from build123d import *

# Parameters (mm, degrees)
F0_R           = 3.75
F1_DEPTH       = 1
F2_R           = 5
F3_R           = 1
F5_DEPTH       = 25
F7_DEPTH       = 25
F8_T1_DEPTH    = 10.2705098312
F10_DEPTH      = 30
F10_DEPTH_BACK = 25


# Not quite as in the source:
# - a fillet or chamfer that OpenCascade refuses, or shapes differently, is made with other operations: its cross-section is extruded or revolved along the edge and cut away or added


with BuildPart() as f1:
    # F0 (on Front) → F1 (new body)
    with BuildSketch(Plane.XZ):
        with BuildLine():
            Line((-27.5, -10), (7.9370479853, -10))
            Line((7.9370479853, -10), (20.3712052174, -7.3570382915))
            ThreePointArc((20.3712052174, -7.3570382915), (25.1669262461, -4.5995427), (27.4438066413, 0.4421373561))
            ThreePointArc((27.4438066413, 0.4421373561), (27.487512587, 1.2231450576), (27.4438066413, 2.004152759))
            ThreePointArc((27.4438066413, 2.004152759), (24.4984425132, 7.7095966656), (18.5, 10))
            Line((18.5, 10), (-12.5, 10))
            Line((-12.5, 10), (-27.5, -10))
        make_face()
        with Locations((18.5, 1.2231450576)):
            Circle(F0_R, mode=Mode.SUBTRACT)
    extrude(amount=F1_DEPTH)

    # F2
    f2_edges = [f1.edges().sort_by_distance(p)[0] for p in [
        (-12.5, -0.5, 10),
    ]]
    fillet(f2_edges, radius=F2_R)

    # F3
    f3_edges = [f1.edges().sort_by_distance(p)[0] for p in [
        (-27.5, -0.5, -10),
    ]]
    fillet(f3_edges, radius=F3_R)

    # F4 (on face) → F5 (cut)
    with BuildSketch(Plane.XZ.offset(1)):
        Polygon((-24.7211863589, -8.9615818119), (-25.5, -10), (-25.5, -14.0343736857), (7.9370479853, -14.0343736857), (8.0576272821, -10), (7.2788136411, -8.9615818119), (6.5, -10), (6.4576272821, -10), (5.6788136411, -8.9615818119), (4.9, -10), (4.8576272821, -10), (4.0788136411, -8.9615818119), (3.3, -10), (3.2576272821, -10), (2.4788136411, -8.9615818119), (1.7, -10), (1.6576272821, -10), (0.8788136411, -8.9615818119), (0.1, -10), (0.0576272821, -10), (-0.7211863589, -8.9615818119), (-1.5, -10), (-1.5423727179, -10), (-2.3211863589, -8.9615818119), (-3.1, -10), (-3.1423727179, -10), (-3.9211863589, -8.9615818119), (-4.7, -10), (-4.7423727179, -10), (-5.5211863589, -8.9615818119), (-6.3, -10), (-6.3423727179, -10), (-7.1211863589, -8.9615818119), (-7.9, -10), (-7.9423727179, -10), (-8.7211863589, -8.9615818119), (-9.5, -10), (-9.5423727179, -10), (-10.3211863589, -8.9615818119), (-11.1, -10), (-11.1423727179, -10), (-11.9211863589, -8.9615818119), (-12.7, -10), (-12.7423727179, -10), (-13.5211863589, -8.9615818119), (-14.3, -10), (-14.3423727179, -10), (-15.1211863589, -8.9615818119), (-15.9, -10), (-15.9423727179, -10), (-16.7211863589, -8.9615818119), (-17.5, -10), (-17.5423727179, -10), (-18.3211863589, -8.9615818119), (-19.1, -10), (-19.1423727179, -10), (-19.9211863589, -8.9615818119), (-20.7, -10), (-20.7423727179, -10), (-21.5211863589, -8.9615818119), (-22.3, -10), (-22.3423727179, -10), (-23.1211863589, -8.9615818119), (-23.9, -10), (-23.9423727179, -10), align=None)
    extrude(amount=-F5_DEPTH, mode=Mode.SUBTRACT)

    # F6 (on face) → F7 (cut)
    with BuildSketch(Plane.XZ.offset(1)):
        Polygon((-26.6561899334, -14.2840119079), (-25.5, -10), (-26.3, -8.4), (-30.4410159588, -7.8742252663), align=None)
    extrude(amount=-F7_DEPTH, mode=Mode.SUBTRACT)

    # F8: fillet of radius 3 on 1 edges, made by hand

    # F8_s2 → F8_t1 (cut)
    with BuildSketch(Plane.XZ.offset(-4.6352549156)):
        with BuildLine():
            ThreePointArc((-25.1875388203, -6.916718427), (-25.7754167621, -8.4473016411), (-25.4708203932, -10.0583592135))
            Line((-25.4708203932, -10.0583592135), (-26.3, -8.4))
            Line((-26.3, -8.4), (-25.1875388203, -6.916718427))
        make_face()
    extrude(amount=F8_T1_DEPTH, mode=Mode.SUBTRACT)

    # F9 (on Right) → F10 (cut, two sides)
    with BuildSketch(Plane.YZ) as f10_sk:
        Polygon((-2.5567745324, -10.8186043799), (-0.4, -10), (-1, -6.9173601342), (-2.5567745324, -6.9173601342), align=None)
    extrude(amount=-F10_DEPTH, mode=Mode.SUBTRACT)
    extrude(f10_sk.sketch, amount=F10_DEPTH_BACK, mode=Mode.SUBTRACT)


solid = f1.part
For this review, take the finished solid that the model builds, in its own axes (mm). Round coordinates to 2 decimals unless told otherwise and drop trailing zeros. Write each loop counter-clockwise with the first axis right and the second up, starting at its lowest first coordinate (ties: lowest second). Pieces come first, ordered by that corner, then holes. Notation, with made-up numbers: (86, 89) - (101, 89) arc R33 cw to (101, 126) - close; hole circle Ø5 at (-34.75, 87). An arc over 180 degrees is marked (long way). Use a Markdown table: item, result.
Q1. We need section B-B (x = 17). Give the boundary of the cut face in (y, z).
Derived:
| item | result |
|---|---|
| outline | (-1, -6.92) - (-0.77, -8.07) - (0, -8.07) - (0, -2.21) - (-1, -2.21) - close; (-1, 4.66) - (0, 4.66) - (0, 10) - (-1, 10) - close |
Q2. We need section A-A (z = 3.5). Give the boundary of the cut face in (x, y) (3 decimals), plus the area to 3 significant figures.
Derived:
| item | result |
|---|---|
| outline | (-17.375, -1) - (15.52, -1) - (15.52, 0) - (-17.375, 0) - close; (21.48, -1) - (27.146, -1) - (27.146, 0) - (21.48, 0) - close |
| area | 38.6 mm2 |
Q3. The part is to be moulded in two halves that separate along X. For faces 1 (the cylindrical face through (14.754, -0.493, 1.388)), 2 (the flat face through (0, 0, 0)), 3 (the cylindrical face through (25.11, -0.49, -4.66)), say which applies: pulls with the +X half, pulls with the -X half, needs draft (parallel to the pull), parting line crosses it, or undercut.
Derived:
| item | result |
|---|---|
| face 1 | undercut |
| face 2 | needs draft |
| face 3 | pulls with the +X half |
Q4. Wall thickness on line 1 along X through (y, z) = (-0.35, 4.25); line 2 along Z through (x, y) = (18.5, -0.55); line 3 along X through (y, z) = (-0.65, 0): over which ranges is each line inside the solid? List them lowest first.
Derived:
| item | result |
|---|---|
| line 1 | x = -16.81 to 16.29, 20.71 to 26.89 |
| line 2 | z = -7.75 to -2.53, 4.97 to 10 |
| line 3 | x = -20 to 14.96, 22.04 to 27.38 |
Q5. We need section C-C (z = 6). Give the boundary of the cut face in (x, y), plus the area to 3 significant figures.
Derived:
| item | result |
|---|---|
| outline | (-15.5, -1) - (25.98, -1) - (25.98, 0) - (-15.5, 0) - close |
| area | 41.5 mm2 |
